from build123d import *

# Parameters (mm, degrees)
SKIZZE1_W                       = 10
SKIZZE1_H                       = 10
SKIZZE1_W_2                     = 8
SKIZZE1_H_2                     = 8
AUFSATZ_LINEAR_AUSTRAGEN1_DEPTH = 30
SKIZZE2_R                       = 1.75
SCHNITT_LINEAR_AUSTRAGEN1_DEPTH = 35
SKIZZE3_R                       = 2.5
SCHNITT_LINEAR_AUSTRAGEN2_DEPTH = 17
FL_CHE_START                    = 27.5
FL_CHE_VERSCHIEBEN1_OUTLINE_W   = 10
FL_CHE_VERSCHIEBEN1_OUTLINE_H   = 10
FL_CHE_VERSCHIEBEN1_OUTLINE_W_2 = 8
FL_CHE_VERSCHIEBEN1_OUTLINE_H_2 = 8
FL_CHE_VERSCHIEBEN1_DEPTH       = 2.5
FL_CHE_VERSCHIEBEN2_OUTLINE_W   = 10
FL_CHE_VERSCHIEBEN2_OUTLINE_H   = 10
FL_CHE_VERSCHIEBEN2_OUTLINE_W_2 = 8
FL_CHE_VERSCHIEBEN2_OUTLINE_H_2 = 8
FL_CHE_VERSCHIEBEN2_DEPTH       = 2.5
VERRUNDUNG1_R                   = 3


# Read off the part's stored shape, not the designer's step: Fläche verschieben1, Fläche verschieben2
with BuildPart() as part:
    # Skizze1 → Aufsatz-Linear austragen1 (new body)
    with BuildSketch(Plane.XY):
        Rectangle(SKIZZE1_W, SKIZZE1_H)
        Rectangle(SKIZZE1_W_2, SKIZZE1_H_2, mode=Mode.SUBTRACT)
    extrude(amount=AUFSATZ_LINEAR_AUSTRAGEN1_DEPTH)

    # Skizze2 → Schnitt-Linear austragen1 (cut)
    with BuildSketch(Plane(origin=(5, 0, 0), x_dir=(0, 0, -1), z_dir=(1, 0, 0))):
        with Locations(Location((-6, 0, 0), (0, 0, 90))):
            Circle(SKIZZE2_R)
        with Locations(Location((-24, 0, 0), (0, 0, 90))):
            Circle(SKIZZE2_R)
    extrude(amount=-SCHNITT_LINEAR_AUSTRAGEN1_DEPTH, mode=Mode.SUBTRACT)

    # Skizze3 → Schnitt-Linear austragen2 (cut)
    with BuildSketch(Plane.XZ.offset(5)):
        with Locations((0, 13.5)):
            Circle(SKIZZE3_R)
    extrude(amount=-SCHNITT_LINEAR_AUSTRAGEN2_DEPTH, mode=Mode.SUBTRACT)

    # Fläche verschieben1 outline → Fläche verschieben1 (cut)
    with BuildSketch(Plane.XY.offset(FL_CHE_START)):
        Rectangle(FL_CHE_VERSCHIEBEN1_OUTLINE_W, FL_CHE_VERSCHIEBEN1_OUTLINE_H)
        Rectangle(FL_CHE_VERSCHIEBEN1_OUTLINE_W_2, FL_CHE_VERSCHIEBEN1_OUTLINE_H_2, mode=Mode.SUBTRACT)
    extrude(amount=FL_CHE_VERSCHIEBEN1_DEPTH, mode=Mode.SUBTRACT)

    # Fläche verschieben2 outline → Fläche verschieben2 (cut)
    with BuildSketch(Plane.XY):
        Rectangle(FL_CHE_VERSCHIEBEN2_OUTLINE_W, FL_CHE_VERSCHIEBEN2_OUTLINE_H)
        Rectangle(FL_CHE_VERSCHIEBEN2_OUTLINE_W_2, FL_CHE_VERSCHIEBEN2_OUTLINE_H_2, mode=Mode.SUBTRACT)
    extrude(amount=FL_CHE_VERSCHIEBEN2_DEPTH, mode=Mode.SUBTRACT)

    # Verrundung1
    # the kernel refuses this fillet: 3 mm, written as the material it takes off along each edge
    with BuildSketch(Plane(origin=(-12.5, -5, 2.5), x_dir=(0, 0, 1), z_dir=(1, 0, 0)), Plane(origin=(12.5, 5, 27.5), x_dir=(0, -1, 0), z_dir=(-1, 0, 0))) as verrundung1_piece_1:
        with BuildLine():
            CenterArc((VERRUNDUNG1_R, -VERRUNDUNG1_R), VERRUNDUNG1_R, 90, 90)
            Line((0, -VERRUNDUNG1_R), (0, 0))
            Line((0, 0), (VERRUNDUNG1_R, 0))
        make_face()
    extrude(amount=25, mode=Mode.SUBTRACT)
    with BuildSketch(Plane(origin=(12.5, 5, 2.5), x_dir=(0, -1, 0), z_dir=(-1, 0, 0)), Plane(origin=(-12.5, -5, 27.5), x_dir=(0, 0, -1), z_dir=(1, 0, 0))) as verrundung1_piece_2:
        with BuildLine():
            CenterArc((VERRUNDUNG1_R, VERRUNDUNG1_R), VERRUNDUNG1_R, 180, 90)
            Line((0, VERRUNDUNG1_R), (0, 0))
            Line((0, 0), (VERRUNDUNG1_R, 0))
        make_face()
    extrude(amount=25, mode=Mode.SUBTRACT)


solid = part.part
Verification items for the finished model (mm, model axes). A direction names the side the tool comes from. Give positions to 0.01 mm unless a question says otherwise; leave off trailing zeros. Loops run counter-clockwise (first coordinate to the right, second up) from the corner with the lowest first, then second, coordinate; pieces in that order, holes last.
1) Depth check by flat-ended pin: pin 1 Ø4 at (y, z) = (0, 24) entering from +X; pin 2 Ø3 at (y, z) = (0, 6) entering from -X. Enter the tip coordinate at first touch or a pass-through.
2) Sectioned sample at D-D, the plane x = -2.75. Enter the section's corners in (y, z), then the cut area to 3 significant figures.
3) Set-up check for faces 1 (the flat face through (0, -4, 17)), 2 (the flat face through (-4.5, 0, 2.5)): record each of +Z, -Z, +X, -X, +Y, -Y from which the full face is reachable in a straight line by a thin tool's end or side.
4) Sectioned sample at B-B, the plane x = 0. Enter the section's corners in (y, z).
5) Sectioned sample at C-C, the plane y = 0. Enter the section's corners in (x, z).
6) Sectioned sample at A-A, the plane z = 24. Enter the section's corners in (x, y).
7) Thickness scan on line 1 along Z through (x, y) = (-4.75, 0); line 2 along X through (y, z) = (3.5, 24.5). Record the ranges inside material, lowest first.
8) Draft check along X on faces 3 (the flat face through (5, 0, 15)), 4 (the flat face through (0, 4, 17)), 5 (the flat face through (0, 5, 17)). Enter one of: pulls with the +X half, pulls with the -X half, needs draft (parallel to the pull), parting line crosses it, or undercut.
Answers:
1. pin 1: stops at x = 5
1. pin 2: passes through
2. outline: (-5, 5.5) arc R3 ccw to (-4, 3.26) - (-4, 26.74) arc R3 ccw to (-5, 24.5) - close; (4, 3.26) arc R3 ccw to (5, 5.5) - (5, 24.5) arc R3 ccw to (4, 26.74) - close
2. area: 44.2 mm2
3. face 1: +Z, -Z
3. face 2: -Z, +X, -X, +Y, -Y
4. outline: (-5, 5.5) arc R3 ccw to (-4, 3.26) - (-4, 11) - (-5, 11) - close; (-5, 16) - (-4, 16) - (-4, 26.74) arc R3 ccw to (-5, 24.5) - close; (4, 3.26) arc R3 ccw to (5, 5.5) - (5, 11) - (4, 11) - close; (4, 16) - (5, 16) - (5, 24.5) arc R3 ccw to (4, 26.74) - close
5. outline: (-5, 2.5) - (-4, 2.5) - (-4, 4.25) - (-5, 4.25) - close; (-5, 7.75) - (-4, 7.75) - (-4, 22.25) - (-5, 22.25) - close; (-5, 25.75) - (-4, 25.75) - (-4, 27.5) - (-5, 27.5) - close; (4, 2.5) - (5, 2.5) - (5, 4.25) - (4, 4.25) - close; (4, 7.75) - (5, 7.75) - (5, 22.25) - (4, 22.25) - close; (4, 25.75) - (5, 25.75) - (5, 27.5) - (4, 27.5) - close
6. outline: (-5, -5) - (5, -5) - (5, -1.75) - (4, -1.75) - (4, -4) - (-4, -4) - (-4, -1.75) - (-5, -1.75) - close; (-5, 1.75) - (-4, 1.75) - (-4, 4) - (4, 4) - (4, 1.75) - (5, 1.75) - (5, 5) - (-5, 5) - close
7. line 1: z = 2.5 to 4.25, 7.75 to 22.25, 25.75 to 27.5
7. line 2: x = -5 to -4, 4 to 5
8. face 3: pulls with the +X half
8. face 4: undercut
8. face 5: needs draft
